CAD build for the part. Positions are in the model's coordinates, mm. Coordinates: 2 decimals unless noted, no trailing zeros. Write each loop counter-clockwise with the first axis right and the second up, starting at its lowest first coordinate (ties: lowest second). Pieces come first, ordered by that corner, then holes.
```python
from build123d import *

# Parameters (mm, degrees)
BOSS_EXTRUDE1_DEPTH   = 74.341091188
F_0_80_TAPPED_HOLE2_D = 1.19126


with BuildPart() as part:
    # Sketch1 → Boss-Extrude1 (new body)
    with BuildSketch(Plane(origin=(0, 0, 0), x_dir=(1, 0, 0), z_dir=(0, 1, 0))):
        with BuildLine():
            Line((0, -42.854004512), (-763.0290048, -42.854004512))
            ThreePointArc((-763.0290048, -42.854004512), (-805.883009312, 0), (-763.0290048, 42.854004512))
            Line((-763.0290048, 42.854004512), (0, 42.854004512))
            ThreePointArc((0, 42.854004512), (42.854004512, 0), (0, -42.854004512))
        make_face()
    extrude(amount=BOSS_EXTRUDE1_DEPTH)

    # #0-80 Tapped Hole2 (through all)
    with Locations(Plane(origin=(0, 74.341091188, 0), x_dir=(1, 0, 0), z_dir=(0, 1, 0))):
        with Locations((9.862991623, 17.879805094), (0, -13.073814135), (-765.853466012, 17.879805094), (-756.473581397, -13.073814135)):
            Hole(F_0_80_TAPPED_HOLE2_D / 2)


solid = part.part
```
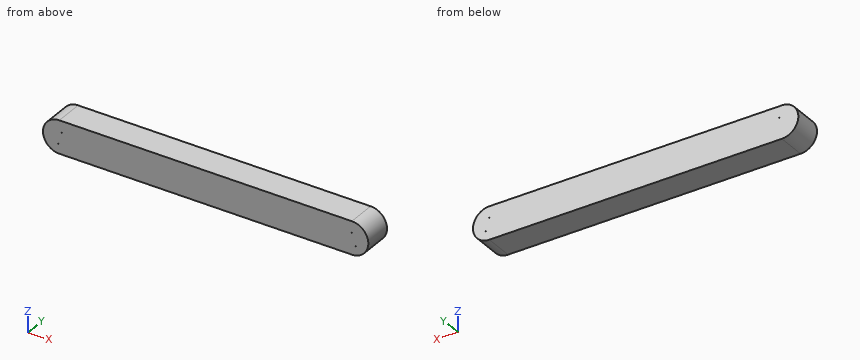
Item 1: Saw through at B-B, the plane z = 33.5. Write the cut outline in (x, y).
Item 2: Flat gauge pins, fed straight in: pin 1 Ø1 at (x, z) = (0, 13.07) entering from -Y; pin 2 Ø4 at (y, z) = (26.5, 27.5) entering from +X; pin 3 Ø5 at (y, z) = (53.5, 21.5) entering from -X. Where does each tip first touch, or does it go through?
Item 3: Wall check: line 1 along X through (y, z) = (21.5, 3); line 2 along X through (y, z) = (65, 13); line 3 along X through (y, z) = (42.5, 2). Give the ranges that are in metal, low to high.
Item 4: Saw through at A-A, the plane y = 21.5. Write the cut outline in (x, z), and give its area (3 significant figures).
Working result:
1. outline: (-789.75, 0) - (26.72, 0) - (26.72, 74.34) - (-789.75, 74.34) - close
2. pin 1: passes through
2. pin 2: stops at x = 34.44
2. pin 3: stops at x = -801.44
3. line 1: x = -805.78 to 42.75
3. line 2: x = -803.86 to -757.06, -755.88 to -0.59, 0.59 to 40.83
3. line 3: x = -805.84 to 42.81
4. outline: (-763.03, -42.85) - (0, -42.85) arc R42.85 ccw to (0, 42.85) - (-763.03, 42.85) arc R42.85 ccw to start; hole circle Ø1.19 at (-765.85, -17.88); hole circle Ø1.19 at (-756.47, 13.07); hole circle Ø1.19 at (0, 13.07); hole circle Ø1.19 at (9.86, -17.88)
4. area: 71,200 mm2
